Source: CAD feature listing. Evaluate the final solid. Frame: model axes, mm. Coordinates: 2 decimals unless noted, no trailing zeros. Order: outer loops, then holes, each group sorted by start corner. A loop starts at its lowest first (then second) coordinate and runs counter-clockwise, first axis right, second up.
```python
from build123d import *

# Parameters (mm, degrees)
EXTRUDE_1_DEPTH            = 2
CUT_EXTRUDE_1_REACH        = 25.67
SKETCH_2_R                 = 1.25
CHAMFER_1_SIZE             = 0.5
CHAMFER_1_OF_MIRROR_3_SIZE = 0.5
CUT_EXTRUDE_5_REACH        = 25.67


with BuildPart() as part:
    # 草图1 → 凸台-拉伸1 (new body)
    with BuildSketch(Plane(origin=(0, 0, 0), x_dir=(1, 0, 0), z_dir=(0, 1, 0))):
        with BuildLine():
            Line((-17, 12.5), (17, 12.5))
            ThreePointArc((17, 12.5), (19.121320344, 11.621320344), (20, 9.5))
            Line((20, 9.5), (20, -9.5))
            ThreePointArc((20, -9.5), (19.121320344, -11.621320344), (17, -12.5))
            Line((17, -12.5), (-17, -12.5))
            ThreePointArc((-17, -12.5), (-19.121320344, -11.621320344), (-20, -9.5))
            Line((-20, -9.5), (-20, 9.5))
            ThreePointArc((-20, 9.5), (-19.121320344, 11.621320344), (-17, 12.5))
        make_face()
    extrude(amount=EXTRUDE_1_DEPTH)

    # 草图2 → 切除-拉伸1 (cut, up to next)
    with BuildSketch(Plane(origin=(0, 2, 0), x_dir=(1, 0, 0), z_dir=(0, 1, 0)), mode=Mode.PRIVATE) as cut_extrude_1_sk1:
        with Locations(Location((-15.75, 0, 0), (0, 0, 270))):
            Circle(SKETCH_2_R)
    cut_extrude_1_tool1 = extrude(cut_extrude_1_sk1.sketch, amount=-CUT_EXTRUDE_1_REACH, mode=Mode.PRIVATE) & part.part
    cut_extrude_1 = cut_extrude_1_tool1.solids().sort_by_distance((-15.75, 2, 0))[0]
    add(cut_extrude_1, mode=Mode.SUBTRACT)

    # 倒角1
    chamfer_1_edges = [part.edges().sort_by_distance(p)[0] for p in [
        (-15.75, 2, -1.25),
    ]]
    chamfer(chamfer_1_edges, length=CHAMFER_1_SIZE)

    # 镜向3: 切除-拉伸1 across plane
    add(cut_extrude_1.mirror(Plane(origin=(0, 0, 0), x_dir=(0, 0, 1), z_dir=(1, 0, 0))), mode=Mode.SUBTRACT)

    # 倒角1 of 镜向3
    chamfer_1_of_mirror_3_edges = [part.edges().sort_by_distance(p)[0] for p in [
        (15.75, 2, -1.25),
    ]]
    chamfer(chamfer_1_of_mirror_3_edges, length=CHAMFER_1_OF_MIRROR_3_SIZE)

    # 草图6 → 切除-拉伸5 (cut, up to next)
    with BuildSketch(Plane(origin=(0, 2, 0), x_dir=(1, 0, 0), z_dir=(0, 1, 0)), mode=Mode.PRIVATE) as cut_extrude_5_sk1:
        with BuildLine():
            Line((-10.036, 3.3), (-7.336, 3.3))
            ThreePointArc((-7.336, 3.3), (-7.053157288, 3.417157288), (-6.936, 3.7))
            Line((-6.936, 3.7), (-6.936, 5.1))
            ThreePointArc((-6.936, 5.1), (-6.818842712, 5.382842712), (-6.536, 5.5))
            Line((-6.536, 5.5), (0.664, 5.5))
            ThreePointArc((0.664, 5.5), (0.946842712, 5.382842712), (1.064, 5.1))
            Line((1.064, 5.1), (1.064, 3.7))
            ThreePointArc((1.064, 3.7), (1.181157288, 3.417157288), (1.464, 3.3))
            Line((1.464, 3.3), (4.164, 3.3))
            ThreePointArc((4.164, 3.3), (4.446842712, 3.182842712), (4.564, 2.9))
            Line((4.564, 2.9), (4.564, 0.5))
            ThreePointArc((4.564, 0.5), (4.446842712, 0.217157288), (4.164, 0.1))
            Line((4.164, 0.1), (-10.036, 0.1))
            ThreePointArc((-10.036, 0.1), (-10.318842712, 0.217157288), (-10.436, 0.5))
            Line((-10.436, 0.5), (-10.436, 2.9))
            ThreePointArc((-10.436, 2.9), (-10.318842712, 3.182842712), (-10.036, 3.3))
        make_face()
    cut_extrude_5_tool1 = extrude(cut_extrude_5_sk1.sketch, amount=-CUT_EXTRUDE_5_REACH, mode=Mode.PRIVATE) & part.part
    # 草图6 → 切除-拉伸5 (cut, up to next)
    with BuildSketch(Plane(origin=(0, 2, 0), x_dir=(1, 0, 0), z_dir=(0, 1, 0)), mode=Mode.PRIVATE) as cut_extrude_5_sk2:
        with BuildLine():
            Line((-10.925, -2.2), (-1.925, -2.2))
            ThreePointArc((-1.925, -2.2), (-1.642157288, -2.317157288), (-1.525, -2.6))
            Line((-1.525, -2.6), (-1.525, -5.1))
            ThreePointArc((-1.525, -5.1), (-1.642157288, -5.382842712), (-1.925, -5.5))
            Line((-1.925, -5.5), (-10.925, -5.5))
            ThreePointArc((-10.925, -5.5), (-11.207842712, -5.382842712), (-11.325, -5.1))
            Line((-11.325, -5.1), (-11.325, -2.6))
            ThreePointArc((-11.325, -2.6), (-11.207842712, -2.317157288), (-10.925, -2.2))
        make_face()
    cut_extrude_5_tool2 = extrude(cut_extrude_5_sk2.sketch, amount=-CUT_EXTRUDE_5_REACH, mode=Mode.PRIVATE) & part.part
    # 草图6 → 切除-拉伸5 (cut, up to next)
    with BuildSketch(Plane(origin=(0, 2, 0), x_dir=(1, 0, 0), z_dir=(0, 1, 0)), mode=Mode.PRIVATE) as cut_extrude_5_sk3:
        with BuildLine():
            Line((0.5, -0.25), (10.3, -0.25))
            ThreePointArc((10.3, -0.25), (10.512132034, -0.337867966), (10.6, -0.55))
            Line((10.6, -0.55), (10.6, -5.2))
            ThreePointArc((10.6, -5.2), (10.512132034, -5.412132034), (10.3, -5.5))
            Line((10.3, -5.5), (0.5, -5.5))
            ThreePointArc((0.5, -5.5), (0.287867966, -5.412132034), (0.2, -5.2))
            Line((0.2, -5.2), (0.2, -0.55))
            ThreePointArc((0.2, -0.55), (0.287867966, -0.337867966), (0.5, -0.25))
        make_face()
    cut_extrude_5_tool3 = extrude(cut_extrude_5_sk3.sketch, amount=-CUT_EXTRUDE_5_REACH, mode=Mode.PRIVATE) & part.part
    add(cut_extrude_5_tool1.solids().sort_by_distance((-2.936, 2, -2.42379))[0], mode=Mode.SUBTRACT)
    add(cut_extrude_5_tool2.solids().sort_by_distance((-6.425, 2, 3.85))[0], mode=Mode.SUBTRACT)
    add(cut_extrude_5_tool3.solids().sort_by_distance((5.4, 2, 2.875))[0], mode=Mode.SUBTRACT)


solid = part.part
```
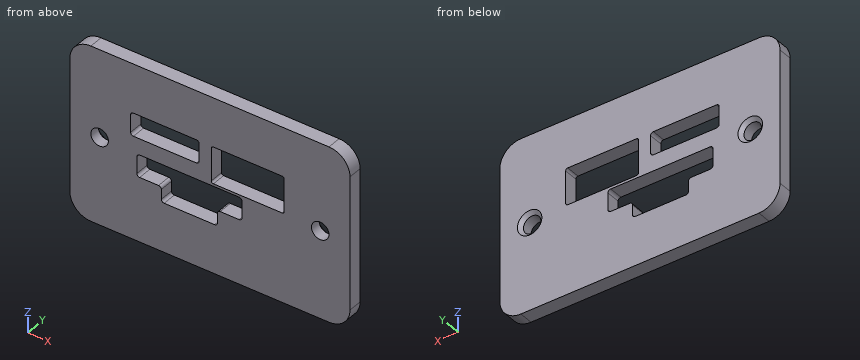
Q1. Section query C-C on x = 8.5. Output: boundary loops of the cut face in (y, z).
Solutions:
outline: (0, -12.5) - (2, -12.5) - (2, 0.25) - (0, 0.25) - close; (0, 5.5) - (2, 5.5) - (2, 12.5) - (0, 12.5) - close
Q2. Material intervals for line 1 along X through (y, z) = (1.15, 0); line 2 along X through (y, z) = (1.1, 3.75) (3 decimals); line 3 along Z through (x, y) = (-6.5, 0.75), sorted ascending.
Solutions:
line 1: x = -20 to -17, -14.5 to 14.5, 17 to 20
line 2: x = -20 to -11.325, -1.525 to 0.2, 10.6 to 20
line 3: z = -12.5 to -5.5, -0.1 to 2.2, 5.5 to 12.5
Q3. Section query A-A on x = -15.75. Output: boundary loops of the cut face in (y, z), plus the area to 4 significant figures.
Solutions:
outline: (0, -12.5) - (2, -12.5) - (2, -1.75) - (1.5, -1.25) - (0, -1.25) - close; (0, 1.25) - (1.5, 1.25) - (2, 1.75) - (2, 12.5) - (0, 12.5) - close
area: 44.75 mm2
Q4. Section query B-B on y = 0.8. Give the number of separate pieces and of enclosed holes in the cut face, plus the area to 3 significant figures.
Solutions:
separate pieces: 1
enclosed holes: 5
area: 830 mm2
